For this review, take the finished solid that the model builds, in its own axes (mm). Face numbers are marked on the shaded views. A direction names the side the tool comes from. Coordinates: 2 decimals unless noted, no trailing zeros. Write each loop counter-clockwise with the first axis right and the second up, starting at its lowest first coordinate (ties: lowest second). Pieces come first, ordered by that corner, then holes.
1) We need section C-C on x = -15. Write out the cut boundary in (y, z), then the cut area to 3 significant figures.
2) We need section D-D on y = -3. Give the number of separate pieces and of enclosed holes in the cut face, then the cut area to 3 significant figures.
3) To check wall thickness, follow line 1 along Z through (x, y) = (15.5, 2.25); line 2 along Z through (x, y) = (-3.5, 3.5); line 3 along X through (y, z) = (2.25, -15.5). State the ranges of each line that lie inside material, in increasing order.
4) We need section B-B on z = -9. Write out the cut boundary in (x, y).
5) For the marked faces 1 and 2, list the 3-axis set-ups (+Z, -Z, +X, -X, +Y, -Y) from which the entire face can be reached by the end or side of a thin tool; tool diameter is ignored.
6) Mouldability with a two-part tool opening along X and no side actions: class the marked faces 3, 4 and 5 as pulls with the +X half, pulls with the -X half, needs draft (parallel to the pull), parting line crosses it, or undercut.
7) We need section A-A on x = 0. Write out the cut boundary in (y, z), then the cut area to 3 significant figures.
8) Insertion check: P1, Ø2.5, axis at y = 0, z = 16.5, coming from the +X side; P2, Ø1.5, axis at y = -1, z = -13.5, coming from the -X side; P3, Ø0.5, axis at x = -7.5, y = -2, coming from the +Z side. Each pin has a flat end and moves straight along its axis. Give the tip position at first contact, or say it passes through.
from build123d import *

# Parameters (mm, degrees)
F0_R     = 5
F1_DEPTH = 5
F3_DEPTH = 10


with BuildPart() as f1:
    # F0 (on Front) → F1 (new body, symmetric)
    with BuildSketch(Plane.XZ):
        with BuildLine():
            Line((-8.043049, 14.587102), (-7.100528, 12.470164))
            ThreePointArc((-7.100528, 12.470164), (-8.365104, 11.659654), (-9.538033, 10.721401))
            Line((-9.538033, 10.721401), (-11.668586, 12.63976))
            ThreePointArc((-11.668586, 12.63976), (-14.247489, 12.452749), (-13.2808, 10.054578))
            Line((-13.2808, 10.054578), (-11.558728, 8.504017))
            ThreePointArc((-11.558728, 8.504017), (-12.384311, 7.24923), (-13.074213, 5.91502))
            Line((-13.074213, 5.91502), (-15.800837, 6.800954))
            ThreePointArc((-15.800837, 6.800954), (-18.080718, 5.581177), (-16.22218, 3.783526))
            Line((-16.22218, 3.783526), (-14.018319, 3.067448))
            ThreePointArc((-14.018319, 3.067448), (-14.262159, 1.585348), (-14.349743, 0.085878))
            Line((-14.349743, 0.085878), (-17.20098, -0.213799))
            ThreePointArc((-17.20098, -0.213799), (-18.787627, -2.255432), (-16.358597, -3.141732))
            Line((-16.358597, -3.141732), (-14.054015, -2.899511))
            ThreePointArc((-14.054015, -2.899511), (-13.673949, -4.352656), (-13.144072, -5.758113))
            Line((-13.144072, -5.758113), (-15.626917, -7.191584))
            ThreePointArc((-15.626917, -7.191584), (-16.245984, -9.702056), (-13.666465, -9.523756))
            Line((-13.666465, -9.523756), (-11.659644, -8.365118))
            ThreePointArc((-11.659644, -8.365118), (-10.72139, -9.538045), (-9.665672, -10.606474))
            Line((-9.665672, -10.606474), (-11.350818, -12.925879))
            ThreePointArc((-11.350818, -12.925879), (-10.895264, -15.471106), (-8.611276, -14.259036))
            Line((-8.611276, -14.259036), (-7.249215, -12.38432))
            ThreePointArc((-7.249215, -12.38432), (-5.915005, -13.07422), (-4.515989, -13.620879))
            Line((-4.515989, -13.620879), (-5.11206, -16.425172))
            ThreePointArc((-5.11206, -16.425172), (-3.660653, -18.565062), (-2.06712, -16.528799))
            Line((-2.06712, -16.528799), (-1.585331, -14.262161))
            ThreePointArc((-1.585331, -14.262161), (-0.085861, -14.349743), (1.414549, -14.28011))
            Line((1.414549, -14.28011), (2.01062, -17.084403))
            ThreePointArc((2.01062, -17.084403), (4.206918, -18.448949), (4.83446, -15.940583))
            Line((4.83446, -15.940583), (4.352671, -13.673944))
            ThreePointArc((4.352671, -13.673944), (5.758128, -13.144066), (7.100499, -12.470181))
            Line((7.100499, -12.470181), (8.785646, -14.789586))
            ThreePointArc((8.785646, -14.789586), (11.347075, -15.142846), (10.900118, -12.596095))
            Line((10.900118, -12.596095), (9.538057, -10.721379))
            ThreePointArc((9.538057, -10.721379), (10.606485, -9.66566), (11.558708, -8.504044))
            Line((11.558708, -8.504044), (14.041553, -9.937515))
            ThreePointArc((14.041553, -9.937515), (16.525219, -9.218407), (15.081047, -7.073628))
            Line((15.081047, -7.073628), (13.074227, -5.914989))
            ThreePointArc((13.074227, -5.914989), (13.620884, -4.515973), (14.018312, -3.067481))
            Line((14.018312, -3.067481), (16.869549, -3.367158))
            ThreePointArc((16.869549, -3.367158), (18.846003, -1.700022), (16.654325, -0.328066))
            Line((16.654325, -0.328066), (14.349743, -0.085845))
            ThreePointArc((14.349743, -0.085845), (14.280109, 1.414566), (14.054022, 2.899478))
            Line((14.054022, 2.899478), (16.780646, 3.785412))
            ThreePointArc((16.780646, 3.785412), (17.908141, 6.112313), (15.34792, 6.474221))
            Line((15.34792, 6.474221), (13.144059, 5.758143))
            ThreePointArc((13.144059, 5.758143), (12.470173, 7.100514), (11.659664, 8.365091))
            Line((11.659664, 8.365091), (13.790217, 10.28345))
            ThreePointArc((13.790217, 10.28345), (13.8738, 12.867773), (11.387719, 12.157057))
            Line((11.387719, 12.157057), (9.665647, 10.606496))
            ThreePointArc((9.665647, 10.606496), (8.504031, 11.558718), (7.249244, 12.384303))
            Line((7.249244, 12.384303), (8.415335, 15.003385))
            ThreePointArc((8.415335, 15.003385), (7.440552, 17.398278), (5.458479, 15.737827))
            Line((5.458479, 15.737827), (4.515958, 13.620889))
            ThreePointArc((4.515958, 13.620889), (3.067464, 14.018315), (1.585364, 14.262157))
            Line((1.585364, 14.262157), (1.585364, 17.129099))
            ThreePointArc((1.585364, 17.129099), (-0.279235, 18.920463), (-1.414582, 16.597383))
            Line((-1.414582, 16.597383), (-1.414582, 14.280107))
            ThreePointArc((-1.414582, 14.280107), (-2.899494, 14.054018), (-4.35264, 13.673954))
            Line((-4.35264, 13.673954), (-5.51873, 16.293037))
            ThreePointArc((-5.51873, 16.293037), (-7.950739, 17.171128), (-8.043049, 14.587102))
        make_face()
        Circle(F0_R, mode=Mode.SUBTRACT)
    extrude(amount=F1_DEPTH, both=True)

    # F2 (on face) → F3 (cut)
    with BuildSketch(Plane.XZ.offset(5)):
        with BuildLine():
            ThreePointArc((-6.336898, 10.013302), (-8.379215, 8.379215), (-10.013302, 6.336898))
            ThreePointArc((-10.013302, 6.336898), (-10.301966, 5.695961), (-10.400791, 5))
            Line((-10.400791, 5), (-4.153312, 5))
            ThreePointArc((-4.153312, 5), (-3.887479, 5.209367), (-3.611111, 5.404616))
            ThreePointArc((-3.611111, 5.404616), (-2.795207, 6.304803), (-2.5, 7.483315))
            Line((-2.5, 7.483315), (-2.5, 7.900791))
            ThreePointArc((-2.5, 7.900791), (-3.794232, 10.090796), (-6.336898, 10.013302))
        make_face()
        with BuildLine():
            Line((-4.153312, 5), (-10.400791, 5))
            ThreePointArc((-10.400791, 5), (-9.668558, 3.232233), (-7.900791, 2.5))
            Line((-7.900791, 2.5), (-7.483315, 2.5))
            ThreePointArc((-7.483315, 2.5), (-6.304803, 2.795207), (-5.404616, 3.611111))
            ThreePointArc((-5.404616, 3.611111), (-4.829156, 4.350776), (-4.153312, 5))
        make_face()
        with BuildLine():
            ThreePointArc((6.336898, 10.013302), (3.794232, 10.090796), (2.5, 7.900791))
            Line((2.5, 7.900791), (2.5, 7.483315))
            ThreePointArc((2.5, 7.483315), (2.795207, 6.304803), (3.611111, 5.404616))
            ThreePointArc((3.611111, 5.404616), (4.596194, 4.596194), (5.404616, 3.611111))
            ThreePointArc((5.404616, 3.611111), (6.304803, 2.795207), (7.483315, 2.5))
            Line((7.483315, 2.5), (7.900791, 2.5))
            ThreePointArc((7.900791, 2.5), (10.090796, 3.794232), (10.013302, 6.336898))
            ThreePointArc((10.013302, 6.336898), (8.379215, 8.379215), (6.336898, 10.013302))
        make_face()
        with BuildLine():
            Line((-7.483315, -2.5), (-7.900791, -2.5))
            ThreePointArc((-7.900791, -2.5), (-10.090796, -3.794232), (-10.013302, -6.336898))
            ThreePointArc((-10.013302, -6.336898), (-8.379215, -8.379215), (-6.336898, -10.013302))
            ThreePointArc((-6.336898, -10.013302), (-3.794232, -10.090796), (-2.5, -7.900791))
            Line((-2.5, -7.900791), (-2.5, -7.483315))
            ThreePointArc((-2.5, -7.483315), (-2.795207, -6.304803), (-3.611111, -5.404616))
            ThreePointArc((-3.611111, -5.404616), (-4.596194, -4.596194), (-5.404616, -3.611111))
            ThreePointArc((-5.404616, -3.611111), (-6.304803, -2.795207), (-7.483315, -2.5))
        make_face()
        with BuildLine():
            ThreePointArc((5.404616, -3.611111), (4.596194, -4.596194), (3.611111, -5.404616))
            ThreePointArc((3.611111, -5.404616), (2.795207, -6.304803), (2.5, -7.483315))
            Line((2.5, -7.483315), (2.5, -7.900791))
            ThreePointArc((2.5, -7.900791), (3.794232, -10.090796), (6.336898, -10.013302))
            ThreePointArc((6.336898, -10.013302), (8.379215, -8.379215), (10.013302, -6.336898))
            ThreePointArc((10.013302, -6.336898), (10.090796, -3.794232), (7.900791, -2.5))
            Line((7.900791, -2.5), (7.483315, -2.5))
            ThreePointArc((7.483315, -2.5), (6.304803, -2.795207), (5.404616, -3.611111))
        make_face()
    extrude(amount=-F3_DEPTH, mode=Mode.SUBTRACT)


solid = f1.part
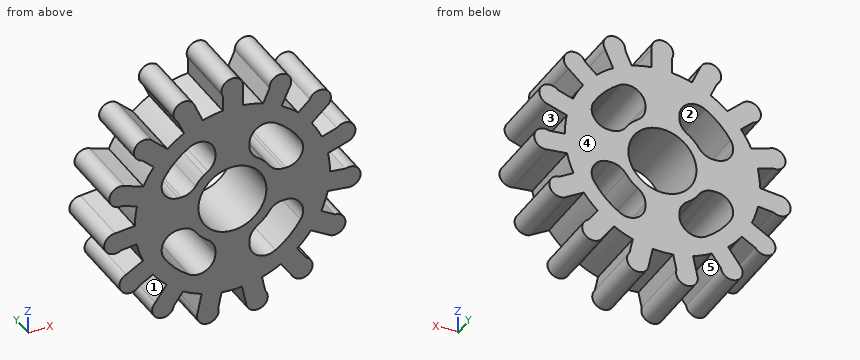
Result:
1. outline: (-5, -10.27) - (5, -10.27) - (5, -6.83) - (-5, -6.83) - close; (-5, -3) - (5, -3) - (5, 0.02) - (-5, 0.02) - close; (-5, 3.39) - (5, 3.39) - (5, 6.54) - (-5, 6.54) - close
1. area: 96.1 mm2
2. separate pieces: 1
2. enclosed holes: 5
2. area: 597 mm2
3. line 1: z = -10.2 to -7.15, -3.22 to -0.21, 3.37 to 6.61
3. line 2: z = -18.56 to -9.9, -5.48 to -3.57, 3.57 to 5.48, 9.9 to 13.92
3. line 3: x = -10.83 to -9.56, -4.92 to -1.85, 1.67 to 4.74, 9.56 to 10.83
4. outline: (-16.59, -5) - (-12.76, -5) - (-12.76, 5) - (-16.59, 5) - close; (-11.18, -5) - (-7.71, -5) - (-7.71, 5) - (-11.18, 5) - close; (-2.75, -5) - (2.75, -5) - (2.75, 5) - (-2.75, 5) - close; (7.71, -5) - (11.18, -5) - (11.18, 5) - (7.71, 5) - close; (12.42, -5) - (16.59, -5) - (16.59, 5) - (12.42, 5) - close
5. face 1: -X, +Y, -Y
5. face 2: +Y, -Y
6. face 3: pulls with the +X half
6. face 4: needs draft
6. face 5: undercut
7. outline: (-5, -14.35) - (5, -14.35) - (5, -5) - (-5, -5) - close; (-5, 5) - (5, 5) - (5, 18.95) - (-5, 18.95) - close
7. area: 233 mm2
8. P1: stops at x = 8.65
8. P2: stops at x = -11.8
8. P3: stops at z = 17.43
